Here's how the part is built. I have some questions about the finished solid (model axes, mm). A direction names the side the tool comes from. Give positions to 0.01 mm unless a question says otherwise; leave off trailing zeros. Write each loop counter-clockwise with the first axis right and the second up, starting at its lowest first coordinate (ties: lowest second). Pieces come first, ordered by that corner, then holes. Notation, with made-up numbers: (-34, 23) - (-19, 23) arc R19 cw to (-19, 44) - close; hole circle Ø5 at (-7.5, 66). An arc over 180 degrees is marked (long way). Use a Markdown table: item, result.
```python
from build123d import *

# Parameters (mm, degrees)
BASPROSKE_W     = 8
BASPROSKE_H     = 10
TOOTHCUT_DEPTH  = 17.248076809
TEETHCUTS_COUNT = 18
TEETHCUTS_ANGLE = 340
BORSKE_R        = 4
BORE_DEPTH      = 50.0000508
KEYSKE_W        = 3
KEYSKE_H        = 5.4
KEYWAY_DEPTH    = 50.0000508
KEYWAY2_COUNT   = 2
KEYWAY2_ANGLE   = 90


with BuildPart() as part:
    # BasProSke → Base-Revolve (revolve)
    with BuildSketch(Plane(origin=(0, 0, 0), x_dir=(1, 0, 0), z_dir=(0, 1, 0)), mode=Mode.PRIVATE) as base_revolve_sk:
        with Locations((4, 5)):
            Rectangle(BASPROSKE_W, BASPROSKE_H)
    revolve(base_revolve_sk.sketch.rotate(Axis((-10, 0, 0), (1, 0, 0)), 180), axis=Axis((-10, 0, 0), (1, 0, 0)))

    # TooCutSke → ToothCut (cut, through all)
    with BuildSketch(Plane(origin=(0, 0, 0), x_dir=(0, 0, -1), z_dir=(1, 0, 0))):
        with BuildLine():
            ThreePointArc((0.510641536, 7.732156635), (0, 7.749), (-0.510641536, 7.732156635))
            ThreePointArc((-0.510641536, 7.732156635), (-0.82619259, 8.907320741), (-1.515208602, 9.910236529))
            ThreePointArc((-1.515208602, 9.910236529), (0, 10.0254), (1.515208602, 9.910236529))
            ThreePointArc((1.515208602, 9.910236529), (0.82619259, 8.907320741), (0.510641536, 7.732156635))
        make_face()
    toothcut = extrude(amount=TOOTHCUT_DEPTH, mode=Mode.SUBTRACT)

    # TeethCuts: ToothCut ×18 about axis
    teethcuts_axis = Axis((-10, 0, 0), (1, 0, 0))
    for i in range(1, TEETHCUTS_COUNT):
        add(toothcut.rotate(teethcuts_axis, i * TEETHCUTS_ANGLE / (TEETHCUTS_COUNT - 1)), mode=Mode.SUBTRACT)

    # BorSke → Bore (cut, symmetric)
    with BuildSketch(Plane(origin=(0, 0, 0), x_dir=(0, 0, -1), z_dir=(1, 0, 0))):
        with Locations(Location((0, 0, 0), (0, 0, 180))):
            Circle(BORSKE_R)
    extrude(amount=BORE_DEPTH, both=True, mode=Mode.SUBTRACT)

    # KeySke → Keyway (cut, symmetric)
    with BuildSketch(Plane(origin=(0, 0, 0), x_dir=(0, 0, -1), z_dir=(1, 0, 0))):
        with Locations((0, 2.7)):
            Rectangle(KEYSKE_W, KEYSKE_H)
    keyway = extrude(amount=KEYWAY_DEPTH, both=True, mode=Mode.SUBTRACT)

    # Keyway2: Keyway ×2 about axis
    keyway2_axis = Axis((0, 0, 0), (-1, 0, 0))
    for i in range(1, KEYWAY2_COUNT):
        add(keyway.rotate(keyway2_axis, i * KEYWAY2_ANGLE / (KEYWAY2_COUNT - 1)), mode=Mode.SUBTRACT)


solid = part.part
```
Item 1: If we section it at B-B, the plane y = 0: Write out the boundary of the cut face in (x, z), plus the area to 3 significant figures.
Values:
| item | result |
|---|---|
| outline | (0, -10) - (8, -10) - (8, -5.4) - (0, -5.4) - close; (0, 4) - (8, 4) - (8, 10) - (0, 10) - close |
| area | 84.8 mm2 |
Item 2: For faces 4 (the cylindrical face through (3.944, 3.868, -6.714)), 5 (the cylindrical face through (3.94, 2.34, -8.6)), 6 (the cylindrical face through (3.944, -8.909, 0.827)), which set-ups out of +Z, -Z, +X, -X, +Y, -Y let a thin tool reach every point of the face, with its end or its side?
Values:
| item | result |
|---|---|
| face 4 | +X, -X |
| face 5 | -Z, +X, -X |
| face 6 | +X, -X, -Y |
Item 3: Will these pins go through, and if not, where does the flat tip stop? pin 1 Ø3 at (x, z) = (7, -6) entering from -Y; pin 2 Ø4 at (x, z) = (5, 5) entering from +Y; pin 3 Ø1.4 at (x, y) = (5.5, 4.5) entering from -Z; pin 4 Ø6 at (y, z) = (-2.5, -4.5) entering from -X.
Values:
| item | result |
|---|---|
| pin 1 | stops at y = -8.78 |
| pin 2 | stops at y = 8.78 |
| pin 3 | stops at z = -7.32 |
| pin 4 | stops at x = 0 |
Item 4: If we section it at C-C, the plane z = 8.25: Write out the boundary of the cut face in (x, y), plus the area to 3 significant figures.
Values:
| item | result |
|---|---|
| outline | (0, -3.75) - (8, -3.75) - (8, -2.13) - (0, -2.13) - close; (0, -0.84) - (8, -0.84) - (8, 0.84) - (0, 0.84) - close; (0, 2.13) - (8, 2.13) - (8, 3.75) - (0, 3.75) - close |
| area | 39.4 mm2 |
Item 5: If we section it at D-D, the plane z = 6: Write out the boundary of the cut face in (x, y).
Values:
| item | result |
|---|---|
| outline | (0, -6.1) - (8, -6.1) - (8, 6.1) - (0, 6.1) - close |
Item 6: I need wall thicknesses on line 1 along Z through (x, y) = (4.5, 0); line 2 along Y through (x, z) = (4.25, 7); line 3 along Z through (x, y) = (1.75, 8.5). Which ranges of each line are inside material? Lowest first, please. Write a range as [from, to].
Values:
| item | result |
|---|---|
| line 1 | z = [-10, -5.4], [4, 10] |
| line 2 | y = [-6.52, -4.8], [-3.45, 3.45], [4.8, 6.52] |
| line 3 | z = [-5.21, -4.31], [-2.28, -0.67], [0.67, 2.28], [4.31, 5.21] |
Item 7: If we section it at A-A, the plane z = 0: Write out the boundary of the cut face in (x, y).
Values:
| item | result |
|---|---|
| outline | (0, -7.75) - (8, -7.75) - (8, -4) - (0, -4) - close; (0, 5.4) - (8, 5.4) - (8, 7.75) - (0, 7.75) - close |
Item 8: Thinking about a two-plate mould opening in Z: for faces 1 (the cylindrical face through (3.94, 2.36, 8.63)), 2 (the flat face through (8, 0, 5)), 3 (the cylindrical face through (4.056, 2.813, -2.844)), which applies, +Z half, -Z half, draft (parallel to the pull), parting line (faces both ways), or undercut?
Values:
| item | result |
|---|---|
| face 1 | +Z half |
| face 2 | draft |
| face 3 | undercut |
